Autodesk Inventor part; units mm, degrees
ref_plane "YZ Plane" through (0, 0, 0) normal (1, 0, 0) x (0, 1, 0)
ref_plane "XZ Plane" through (0, 0, 0) normal (0, 1, 0) x (-1, 0, 0)
ref_plane "XY Plane" through (0, 0, 0) normal (0, 0, 1) x (1, 0, 0)
sketch "Sketch1" plane through (0, 0, 0) normal (0, 1, 0) x (-1, 0, 0)
  line L0 (-55.6, 105) -> (55.6, 105)
  line L1 (55.6, 105) -> (55.6, -105)
  line L2 (55.6, -105) -> (-55.6, -105)
  line L3 (-55.6, -105) -> (-55.6, 105)
  line L4 (-55.6, 105) -> (55.6, -105) construction
  line L5 (55.6, 105) -> (-55.6, -105) construction
  line L6 (55.6, -105) -> (-15.6, -105)
  line L7 (-15.6, -105) -> (-15.6, -95)
  line L8 (-15.6, -95) -> (55.6, -95)
  line L9 (55.6, -95) -> (55.6, -105)
  line L10 (55.6, 105) -> (45.6, 105)
  line L11 (45.6, 105) -> (45.6, 95)
  line L12 (49.6, 91) -> (55.6, 91)
  line L13 (55.6, 91) -> (55.6, 105)
  arc A0 (45.6, 95) -> (49.6, 91) centre (49.6, 95) ccw
  point P0 (0, 0)
  point P1 (-15.6, -105)
  point P2 (55.6, -95)
  point P3 (55.6, 91)
  dimension "d0" = 111.2
  dimension "d1" = 210
  dimension "d84" = 10
  dimension "d85" = 40
  dimension "d86" = 14
  dimension "d87" = 10
  dimension "d88" = 4
extrude "Extrusion1" add sketch "Sketch1" along normal blind 5 contours L0 L11 A0 L12 L1 L8 L7 L2 L3
sketch "Sketch2" plane through (0, 5, 0) normal (0, 1, 0) x (1, 0, 0)
  line L0 (36, 32.5) -> (-43.6, 32.5) construction
  line L1 (-43.6, -77.5) -> (36, -77.5) construction
  line L2 (-55.6, 95) -> (-55.6, -91) construction
  line L3 (-45.6, -105) -> (55.6, -105)
  point P0 (0, 0)
  point P1 (-12.6, -77.5)
  point P2 (-12.6, 32.5)
  dimension "d6" = 31
  dimension "d7" = 31
  dimension "d17" = 12
  dimension "d18" = 12
  dimension "d89" = 110
  dimension "d90" = 27.5
hole "Hole1" at (-43.6, 5, 77.5) at (-43.6, 5, -32.5) at (-12.6, 5, 77.5) at (-12.6, 5, -32.5) direction (0, -1, 0) diameter 3.8 end through all
sketch "Sketch6" plane through (0, 5, 0) normal (0, 1, 0) x (1, 0, 0)
  line L0 (25.9, 93.5) -> (-42.1, 93.5)
  line L1 (-42.1, 93.5) -> (-42.1, -53.5)
  line L2 (-42.1, -53.5) -> (25.9, -53.5)
  line L3 (25.9, -53.5) -> (25.9, 93.5)
  line L4 (25.9, 93.5) -> (-42.1, -53.5) construction
  line L5 (-42.1, 93.5) -> (25.9, -53.5) construction
  line L6 (55.6, -105) -> (55.6, 105)
  line L7 (-45.6, -105) -> (55.6, -105)
  line L8 (55.6, 105) -> (15.6, 105)
  point P0 (0, 0)
  point P1 (-8.1, 20)
  dimension "d29" = 68
  dimension "d30" = 147
  dimension "d32" = 29.7
  dimension "d91" = 51.5
  dimension "d92" = 11.5
hole "Hole2" at (25.9, 5, -93.5) at (25.9, 5, 53.5) direction (0, -1, 0) diameter 3.8 end through all
sketch "Sketch14" plane through (0, 5, 0) normal (0, 1, 0) x (1, 0, 0)
  line L0 (49.1, 119.5954) -> (49.1, -116.5639) construction
  line L1 (55.6, -105) -> (55.6, 105) construction
  line L2 (-45.6, -105) -> (55.6, -105) construction
  point P0 (0, 0)
  point P1 (49.1, 70)
  point P2 (49.1, -10)
  point P3 (49.1, -90)
  dimension "d93" = 6.5
  dimension "d94" = 15
  dimension "d95" = 80
  dimension "d96" = 80
hole "Hole5" at (49.1, 5, -70) at (49.1, 5, 10) at (49.1, 5, 90) direction (0, -1, 0) diameter 3.8 end through all
sketch "Sketch13" plane through (0, 5, 0) normal (0, 1, 0) x (1, 0, 0)
  line L0 (25.9, 3) -> (25.9, -107.0389) construction
  circle A0 centre (25.9, 93.5) radius 1.9 construction
  circle A1 centre (25.9, -53.5) radius 1.9 construction
  circle A2 centre (-12.6, -77.5) radius 1.9 construction
  circle A3 centre (-43.6, -77.5) radius 1.9 construction
  circle A4 centre (-43.6, 32.5) radius 1.9 construction
  circle A5 centre (-12.6, 32.5) radius 1.9 construction
  line L1 (-55.6, 95) -> (-55.6, -91) construction
  line L2 (55.6, 1.7) -> (26.4, 1.7)
  line L3 (25.9, 2.2) -> (25.9, 3.5)
  line L4 (26.4, 3.5) -> (55.6, 3.5)
  line L5 (55.6, 3.5) -> (55.6, 1.7)
  arc A6 (26.4, 3.5) -> (25.9, 3) centre (26.4, 3) ccw
  arc A7 (25.9, 2.2) -> (26.4, 1.7) centre (26.4, 2.2) ccw
  line L6 (55.6, 105) -> (15.6, 105)
  line L7 (15.6, 105) -> (15.6, 95)
  line L8 (15.6, 95) -> (-55.6, 95)
  line L9 (-55.6, -91) -> (-49.6, -91)
  arc A8 (-45.6, -95) -> (-49.6, -91) centre (-49.6, -95) ccw
  line L10 (-45.6, -95) -> (-45.6, -105)
  line L11 (-45.6, -105) -> (55.6, -105)
  line L12 (55.6, -105) -> (55.6, 105)
  point P0 (0, 0)
  point P1 (25.9, 3)
  dimension "d75" = 1.8
  dimension "d76" = 0.5
  dimension "d77" = 90
  dimension "d78" = 57
extrude "Extrusion9" cut sketch "Sketch13" against normal through all
sketch "Sketch15" plane through (0, 5, 0) normal (0, 1, 0) x (1, 0, 0)
  line L0 (-18.1, -3.5) -> (7.9, -3.5) construction
  line L1 (7.9, -3.5) -> (7.9, -52.5) construction
  line L2 (7.9, -52.5) -> (-18.1, -52.5) construction
  line L3 (-18.1, -52.5) -> (-18.1, -3.5) construction
  circle A0 centre (-12.6, -77.5) radius 1.9 construction
  circle A1 centre (25.9, -53.5) radius 1.9 construction
  point P0 (0, 0)
  dimension "d104" = 26
  dimension "d105" = 49
  dimension "d106" = 25
  dimension "d107" = 18
hole "Hole6" at (-18.1, 5, 3.5) at (7.9, 5, 3.5) at (7.9, 5, 52.5) at (-18.1, 5, 52.5) direction (0, -1, 0) diameter 3.8 end through all
sketch "Sketch16" plane through (0, 5, 0) normal (0, 1, 0) x (1, 0, 0)
  line L0 (-55.6, 95) -> (-55.6, -91)
  line L1 (-55.6, 95) -> (15.6, 95)
  line L2 (15.6, 95) -> (15.6, 77)
  line L3 (15.6, 77) -> (-55.6, 77)
  line L4 (-55.6, 77) -> (-55.6, 95)
  line L5 (15.6, 105) -> (15.6, 95)
  circle A0 centre (38.5, 86.3) radius 7.5
  line L6 (55.6, 105) -> (15.6, 105)
  line L7 (55.6, 3.5) -> (55.6, 105)
  point P0 (0, 0)
  dimension "d115" = 18
  dimension "d116" = 15
  dimension "d117" = 18.7
  dimension "d118" = 17.1
extrude "Extrusion10" cut sketch "Sketch16" against normal through all
fillet "Fillet1" radius 4 2 edges at (15.6, 2.5, -77) (15.6, 2.5, -105)
properties part number "Inner Top Plate"
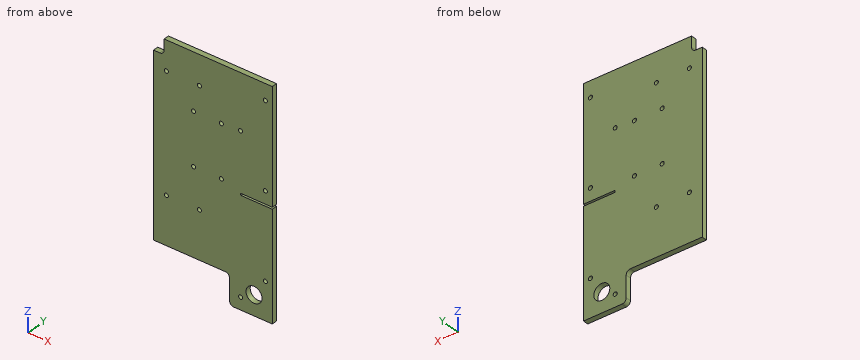
Build history of the part. All positions in model axes, mm. Give positions to 0.01 mm unless a question says otherwise; leave off trailing zeros. Loops run counter-clockwise (first coordinate to the right, second up) from the corner with the lowest first, then second, coordinate; pieces in that order, holes last.
Item 1: Slice it at B-B, the plane y = 3.95. Give the number of separate pieces and of enclosed holes in the cut face, and give its area (3 significant figures).
Answers follow:
separate pieces: 1
enclosed holes: 14
area: 20,800 mm2
Item 2: Drill centre lines: line 1 (X direction, y = 3.7, z = 3.5); line 2 (Z direction, x = 7.9, y = 2); line 3 (X direction, y = 2.15, z = 90). Where is each one in solid material? Low to high.
Answers follow:
line 1: x = -55.6 to -20, -16.2 to 6, 9.8 to 55.6
line 2: z = -77 to 1.6, 5.4 to 50.6, 54.4 to 105
line 3: x = -55.6 to 47.2, 51 to 55.6
Item 3: Slice it at A-A, the plane z = -86.3. List the corners of the cut face in (x, y).
Answers follow:
outline: (15.6, 0) - (31, 0) - (31, 5) - (15.6, 5) - close; (46, 0) - (55.6, 0) - (55.6, 5) - (46, 5) - close
Item 4: Flat gauge pins, fed straight in: pin 1 (2.5 mm diameter, centred on x = 49.1, z = 10, fed in from -Y); pin 2 (2 mm diameter, centred on x = -10.5, y = 2, fed in from -Z); pin 3 (2.5 mm diameter, centred on y = 3.5, z = -88.5, fed in from -X). Where does each tip first touch, or does it go through?
Answers follow:
pin 1: passes through
pin 2: stops at z = -77
pin 3: stops at x = 15.6
Item 5: Slice it at C-C, the plane x = 34.5. List the corners of the cut face in (y, z).
Answers follow:
outline: (0, -105) - (5, -105) - (5, -92.64) - (0, -92.64) - close; (0, -79.96) - (5, -79.96) - (5, -3.5) - (0, -3.5) - close; (0, -1.7) - (5, -1.7) - (5, 105) - (0, 105) - close
